```python
from build123d import *

# Parameters (mm, degrees)
SKETCH1_W           = 155.58
SKETCH1_H           = 155.58
BOSS_EXTRUDE1_DEPTH = 145
CUT_EXTRUDE1_REACH  = 228.454
CUT_EXTRUDE2_DEPTH  = 155.8
SKETCH4_W           = 18
SKETCH4_H           = 18
CUT_EXTRUDE3_DEPTH  = 80
FILLET1_R           = 10
SKETCH5_W           = 18
SKETCH5_H           = 110
CUT_EXTRUDE4_DEPTH  = 10
SKETCH6_W           = 110
SKETCH6_H           = 146
CUT_EXTRUDE5_DEPTH  = 10


with BuildPart() as part:
    # Sketch1 → Boss-Extrude1 (new body)
    with BuildSketch(Plane(origin=(0, 0, 0), x_dir=(1, 0, 0), z_dir=(0, 1, 0))):
        Rectangle(SKETCH1_W, SKETCH1_H)
    extrude(amount=BOSS_EXTRUDE1_DEPTH)

    # Sketch2 → Cut-Extrude1 (cut, up to next)
    with BuildSketch(Plane.XY.offset(77.79), mode=Mode.PRIVATE) as cut_extrude1_sk1:
        with BuildLine():
            Line((43.823001254, 90), (-46.176998746, 90))
            ThreePointArc((-46.176998746, 90), (-53.248066558, 87.071067812), (-56.176998746, 80))
            Line((-56.176998746, 80), (-56.176998746, 8))
            Line((-56.176998746, 8), (-51.176998746, 8))
            Line((-51.176998746, 8), (-51.176998746, 0))
            Line((-51.176998746, 0), (48.823001254, 0))
            Line((48.823001254, 0), (48.823001254, 8))
            Line((48.823001254, 8), (53.823001254, 8))
            Line((53.823001254, 8), (53.823001254, 80))
            ThreePointArc((53.823001254, 80), (50.894069065, 87.071067812), (43.823001254, 90))
        make_face()
    cut_extrude1_tool1 = extrude(cut_extrude1_sk1.sketch, amount=-CUT_EXTRUDE1_REACH, mode=Mode.PRIVATE) & part.part
    add(cut_extrude1_tool1.solids().sort_by_distance((-1.176999, 45.147739, 77.79))[0], mode=Mode.SUBTRACT)

    # Sketch3 → Cut-Extrude2 (cut)
    with BuildSketch(Plane(origin=(77.79, 0, 0), x_dir=(0, 0, -1), z_dir=(1, 0, 0))):
        with BuildLine():
            Line((-55, 80), (-55, 10))
            Line((-55, 10), (55, 10))
            Line((55, 10), (55, 80))
            ThreePointArc((55, 80), (52.071067812, 87.071067812), (45, 90))
            Line((45, 90), (-45, 90))
            ThreePointArc((-45, 90), (-52.071067812, 87.071067812), (-55, 80))
        make_face()
    extrude(amount=-CUT_EXTRUDE2_DEPTH, mode=Mode.SUBTRACT)

    # Sketch4 → Cut-Extrude3 (cut)
    with BuildSketch(Plane.XZ):
        with Locations((62.823001254, -64)):
            Rectangle(SKETCH4_W, SKETCH4_H)
        with Locations((-65.176998746, -64)):
            Rectangle(SKETCH4_W, SKETCH4_H)
        with Locations((62.823001254, 64)):
            Rectangle(SKETCH4_W, SKETCH4_H)
        with Locations((-65.176998746, 64)):
            Rectangle(SKETCH4_W, SKETCH4_H)
    extrude(amount=-CUT_EXTRUDE3_DEPTH, mode=Mode.SUBTRACT)

    # Fillet1
    fillet1_edges = [part.edges().sort_by_distance(p)[0] for p in [
        (-77.79, 145, 0),
        (0, 145, 77.79),
        (77.79, 145, 0),
        (0, 145, -77.79),
    ]]
    fillet(fillet1_edges, radius=FILLET1_R)

    # Sketch5 → Cut-Extrude4 (cut)
    with BuildSketch(Plane.XZ):
        with Locations((-65.176998746, 0)):
            Rectangle(SKETCH5_W, SKETCH5_H)
        with Locations((62.823001254, 0)):
            Rectangle(SKETCH5_W, SKETCH5_H)
    extrude(amount=-CUT_EXTRUDE4_DEPTH, mode=Mode.SUBTRACT)

    # Sketch6 → Cut-Extrude5 (cut)
    with BuildSketch(Plane.XZ):
        with Locations((-1.176998746, 0)):
            Rectangle(SKETCH6_W, SKETCH6_H)
    extrude(amount=-CUT_EXTRUDE5_DEPTH, mode=Mode.SUBTRACT)


solid = part.part
```
Geometry check sheet. Reference: the model listing, model coordinates, mm. A direction names the side the tool comes from. Coordinates: 2 decimals unless noted, no trailing zeros. Loops run counter-clockwise (first coordinate to the right, second up) from the corner with the lowest first, then second, coordinate; pieces in that order, holes last. Notation, with made-up numbers: (42.25, 16.25) -> (61.25, 16.25) arc R32 ccw to (61.25, 46.25) -> close; hole circle Ø5 at (77, 38). An arc over 180 degrees is marked (long way). Put each result on its own line as item: value.
1) Cross-section at A-A on z = 9. Record the boundary of the cut face in (x, y).
Result set:
outline: (-77.79, 0) -> (-74.18, 0) -> (-74.18, 10) -> (-77.79, 10) -> close; (-77.79, 90) -> (77.79, 90) -> (77.79, 135) arc R10 ccw to (67.79, 145) -> (-67.79, 145) arc R10 ccw to (-77.79, 135) -> close; (71.82, 0) -> (77.79, 0) -> (77.79, 10) -> (71.82, 10) -> close
2) Thickness scan on line 1 (Z direction, x = -56.5, y = 71); line 2 (Y direction, x = 0.5, z = -46); line 3 (Z direction, x = 64, y = 89). Record the ranges inside material, lowest first.
Result set:
line 1: z = -77.79 to -73, 73 to 77.79
line 2: y = 90 to 145
line 3: z = -77.79 to -49.36, 49.36 to 77.79
3) Cross-section at D-D on x = 59. Record the boundary of the cut face in (y, z).
Result set:
outline: (0, -77.79) -> (135, -77.79) arc R10 ccw to (145, -67.79) -> (145, 67.79) arc R10 ccw to (135, 77.79) -> (0, 77.79) -> (0, 73) -> (80, 73) -> (80, 55) arc R10 cw to (90, 45) -> (90, -45) arc R10 cw to (80, -55) -> (80, -73) -> (0, -73) -> close
4) Gauge pin test, flat ends, axial feed: pin 1 Ø4 at (x, z) = (50.5, 75.5) entering from +Y; pin 2 Ø5.5 at (x, z) = (-54, -76) entering from +Y; pin 3 Ø6 at (x, z) = (-19, -41.5) entering from -Y. Record the tip position at first contact, or that the pin passes through.
Result set:
pin 1: stops at y = 143.21
pin 2: stops at y = 143.38
pin 3: stops at y = 90
5) Cross-section at C-C on z = -63. Record the boundary of the cut face in (x, y), plus the area to 3 significant figures.
Result set:
outline: (-77.79, 0) -> (-74.18, 0) -> (-74.18, 80) -> (-56.18, 80) arc R10 cw to (-46.18, 90) -> (43.82, 90) arc R10 cw to (53.82, 80) -> (71.82, 80) -> (71.82, 0) -> (77.79, 0) -> (77.79, 135) arc R10 ccw to (67.79, 145) -> (-67.79, 145) arc R10 ccw to (-77.79, 135) -> close
area: 9,780 mm^2
6) Cross-section at B-B on y = 18.5. Record the boundary of the cut face in (x, z).
Result set:
outline: (-77.79, -77.79) -> (-56.18, -77.79) -> (-56.18, -73) -> (-74.18, -73) -> (-74.18, -55) -> (-77.79, -55) -> close; (-77.79, 55) -> (-74.18, 55) -> (-74.18, 73) -> (-56.18, 73) -> (-56.18, 77.79) -> (-77.79, 77.79) -> close; (53.82, -77.79) -> (77.79, -77.79) -> (77.79, -55) -> (71.82, -55) -> (71.82, -73) -> (53.82, -73) -> close; (53.82, 73) -> (71.82, 73) -> (71.82, 55) -> (77.79, 55) -> (77.79, 77.79) -> (53.82, 77.79) -> close
7) Release check for a two-part mould opening along Y. For faces 5 (the cylindrical face through (1.09, 141.99, 74.94)), 6 (the flat face through (71.823, 7, -6)), 7 (the flat face through (-56.177, 45, 75)) record: released by +Y, released by -Y, zero draft, split by the parting line, or undercut.
Result set:
face 5: released by +Y
face 6: zero draft
face 7: undercut
8) Tool access check on faces 1 (the flat face through (-56.177, 45, -75)), 2 (the flat face through (75, 45, 55)), 3 (the flat face through (63, 80, 64)), 4 (the flat face through (-51.177, 4, -75)). Record the directions out of +Z, -Z, +X, -X, +Y, -Y that give a thin tool (end or side, any length) a straight path to the whole face; none if there is none.
Result set:
face 1: +Z, -Z
face 2: +X, -X
face 3: -Y
face 4: +Z, -Z, -Y
